from build123d import *

# Parameters (mm, degrees)
F1_FACE1_R   = 80.9498
F1_FACE1_R_2 = 5.08
F3_DEPTH     = 25.4
F4_R         = 2.54
F5_W         = 12.827
F5_H         = 6.731
F6_DEPTH     = 5.08


with BuildPart() as f1:
    # F0 (on Front) → F1 (revolve)
    with BuildSketch(Plane.XZ):
        Polygon((80.9498, 0), (5.08, 0), (5.08, -10.16), (92.6526099873, -10.16), (92.6526099873, 1.27), (87.5726099873, 1.27), (87.5726099873, -3.81), (86.0298, -3.81), (86.0298, 1.27), (80.9498, 1.27), align=None)
    revolve(axis=Axis((0, 0, -1.5273375125), (0, 0, -1)))

    # F2 (on face) + F1_face1 (on face) → F3 (cut)
    with BuildSketch(Plane(origin=(0, 0, -10.16), x_dir=(1, 0, 0), z_dir=(0, 0, -1))):
        with BuildLine():
            ThreePointArc((80.3791177001, -3.175), (56.8809422709, 56.8809422709), (-3.175, 80.3791177001))
            ThreePointArc((-3.175, 80.3791177001), (-56.8809422709, 56.8809422709), (-80.3791177001, 3.175))
            ThreePointArc((-80.3791177001, 3.175), (-59.0816832218, -54.5915551612), (-3.175, -80.3791177001))
            ThreePointArc((-3.175, -80.3791177001), (-1.5878093455, -80.4261278984), (0, -80.4418))
            ThreePointArc((0, -80.4418), (55.7471096661, -57.9926111769), (80.3791177001, -3.175))
        make_face()
    with BuildSketch(Plane.XY):
        Circle(F1_FACE1_R)
        Circle(F1_FACE1_R_2, mode=Mode.SUBTRACT)
    extrude(amount=-F3_DEPTH, dir=(0, 0, -1), mode=Mode.SUBTRACT)

    # F4
    f4_edges = [f1.edges().sort_by_distance(p)[0] for p in [
        (3.175, 80.379118, -10.16),
        (-92.65261, 0, -10.16),
    ]]
    fillet(f4_edges, radius=F4_R)

    # F5 (on face) → F6 (cut)
    with BuildSketch(Plane.XY.offset(1.27)):
        with Locations((0, 86.5632)):
            Rectangle(F5_W, F5_H)
        Polygon((-83.5453956435, 33.8890975493), (-87.5091566304, 21.6898956148), (-81.1075952192, 19.6099022256), (-77.1438342323, 31.8091041602), align=None)
        Polygon((-58.0473941113, -68.9840858665), (-47.6701331244, -76.5236072976), (-43.7137505912, -71.0781139085), (-54.0910115781, -63.5385924773), align=None)
        Polygon((47.6701331244, -76.5236072976), (58.0473941113, -68.9840858665), (54.0910115781, -63.5385924773), (43.7137505912, -71.0781139085), align=None)
        Polygon((87.5091566304, 21.6898956148), (83.5453956435, 33.8890975493), (77.1438342323, 31.8091041602), (81.1075952192, 19.6099022256), align=None)
    extrude(amount=-F6_DEPTH, mode=Mode.SUBTRACT)


with BuildPart() as f7_1:
    # F7: copy of F1
    add(f1.part)


solid = f1.part
The listing builds one solid part. Answer for the finished solid, in the listing's coordinates (mm). A direction names the side the tool comes from. Coordinates: 2 decimals unless noted, no trailing zeros.
1) Flat-ended cylindrical pins translate along their axes: pin 1 Ø2 at (y, z) = (14.5, -9) entering from +X; pin 2 Ø4 at (x, z) = (2, -1) entering from -Y; pin 3 Ø2 at (y, z) = (50.5, -3.5) entering from -X. Find the tip coordinate at first contact, or state that the pin passes through.
2) Find the intervals of material crossed by L1, parallel to X at y = 0, z = 1.05; L2, parallel to Y at x = 61.5, z = -0.25; L3, parallel to X at y = -42.5, z = -1.5, in increasing order.
3) Determine the mould class of faces 3 (the face through (-85.5, 27.87, -1.23)), 4 (the face through (-12.062, -91.864, -3.113)), 5 (the face through (31, 76, 1.27)) for opening direction Y: pulls with the +Y half, pulls with the -Y half, needs draft (parallel to the pull), parting line crosses it, or undercut.
4) A tool of negligible diameter and unlimited length cuts with its end or side. For faces 1 (the face through (-40, 73, -10.16)), 2 (the face through (79.1, 25.79, -1.23)), from which of +Z, -Z, +X, -X, +Y, -Y can it reach the whole face along a straight path? Write none if from no direction.
Values:
1. pin 1: stops at x = 91.54
1. pin 2: stops at y = -92.65
1. pin 3: stops at x = -78.32
2. L1: x = -92.65 to -87.57, -86.03 to -80.95, 80.95 to 86.03, 87.57 to 92.65
2. L2: y = -69.3 to -62.34, -60.16 to -51.85, 51.85 to 60.16, 62.34 to 69.3
2. L3: x = -82.33 to -76.57, -74.8 to -68.3, 68.3 to 74.8, 76.57 to 82.33
3. face 3: undercut
3. face 4: parting line crosses it
3. face 5: needs draft
4. face 1: -Z, +X, -X, +Y, -Y
4. face 2: +Z
